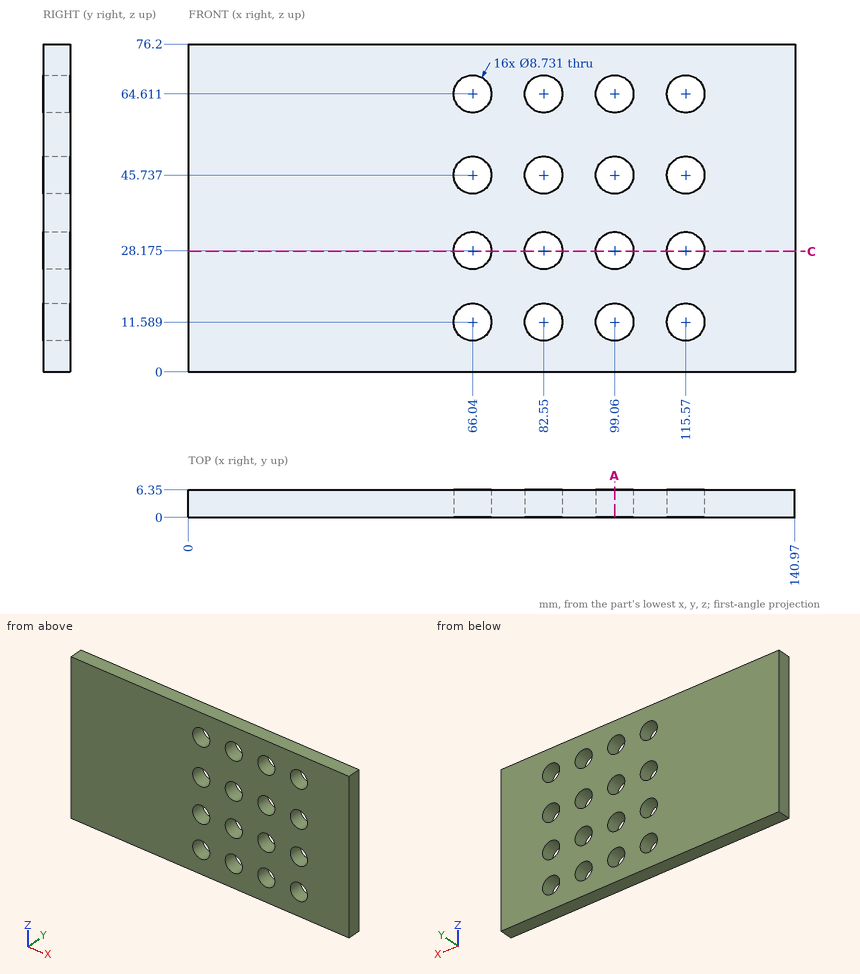
The figure shows three views and two pictorial views of one solid part (mm, origin at its lowest corner). Answer the questions. Give positions to 0.01 mm unless a question says otherwise; leave off trailing zeros. Write each loop counter-clockwise with the first axis right and the second up, starting at its lowest first coordinate (ties: lowest second). Pieces come first, ordered by that corner, then holes.
Q1. Straight lines are drawn through the part: L1, parallel to X at y = 3, z = 11.5 (1 decimal); L2, parallel to X at y = 2.25, z = 10.5; L3, parallel to Z at x = 66.5, y = 6.25 (1 decimal). For each, find the intervals that lie inside material, in ascending order.
Answer:
L1: x = 0 to 61.7, 70.4 to 78.2, 86.9 to 94.7, 103.4 to 111.2, 119.9 to 141
L2: x = 0 to 61.81, 70.27 to 78.32, 86.78 to 94.83, 103.29 to 111.34, 119.8 to 140.97
L3: z = 0 to 7.2, 15.9 to 23.8, 32.5 to 41.4, 50.1 to 60.3, 69 to 76.2
Q2. The part is cut by section C-C on z = 28. Give the vertices of the cut face in (x, y).
Answer:
outline: (0, 0) - (61.68, 0) - (61.68, 6.35) - (0, 6.35) - close; (70.4, 0) - (78.19, 0) - (78.19, 6.35) - (70.4, 6.35) - close; (86.91, 0) - (94.7, 0) - (94.7, 6.35) - (86.91, 6.35) - close; (103.42, 0) - (111.21, 0) - (111.21, 6.35) - (103.42, 6.35) - close; (119.93, 0) - (140.97, 0) - (140.97, 6.35) - (119.93, 6.35) - close
Q3. The part is cut by section A-A on x = 99.06. State how many separate pieces and enclosed holes the cut face has, and give its area (3 significant figures).
Answer:
separate pieces: 5
enclosed holes: 0
area: 262 mm2
